Autodesk Fusion 360 part; units mm, degrees
sketch "Sketch1" plane through (0, 0, 0) normal (0, 0, 1) x (1, 0, 0)
  line L0 (0, 0) -> (100, 0)
  line L1 (100, 0) -> (100, 25)
  line L2 (100, 25) -> (0, 25)
  line L3 (0, 25) -> (0, 0)
  line L4 (0, 25) -> (100, 25)
  line L5 (100, 25) -> (100, 19)
  line L6 (100, 19) -> (0, 19)
  line L7 (0, 19) -> (0, 25)
  circle A0 centre (50, 10) radius 2
  circle A1 centre (10, 10) radius 2
  circle A2 centre (90, 10) radius 2
  dimension "d1" = 100
  dimension "d2" = 6
  dimension "d12" = 4
  dimension "d13" = 4
  dimension "d14" = 4
extrude "Extrude1" add sketch "Sketch1" along normal blind 4 contours L0 L1 L3 L6
extrude "Extrude2" add sketch "Sketch1" along normal blind 9 contours L1 L2 L3 L4 L5 L6 L7
sketch "Sketch2" plane through (0, 0, 9) normal (0, 0, 1) x (1, 0, 0)
  line L0 (0, 19) -> (100, 19)
  line L1 (100, 19) -> (100, 25)
  line L2 (100, 25) -> (0, 25)
  line L3 (0, 25) -> (0, 19)
  line L4 (0, 19) -> (100, 19)
  line L5 (100, 19) -> (100, 44)
  line L6 (100, 44) -> (0, 44)
  line L7 (0, 44) -> (0, 19)
  dimension "d7" = 25
  dimension "d8" = 100
extrude "Extrude3" add sketch "Sketch2" along normal blind 4
fillet "Fillet1" radius 2 13 edges at (50, 44, 13) (0, 31.5, 13) (100, 44, 11) (100, 31.5, 13) (50, 19, 13) (100, 19, 8.5) (100, 9.5, 4) (50, 0, 4) (0, 9.5, 4) (100, 0, 2) (0, 0, 2) (0, 19, 8.5) (0, 44, 11)
Could you check a few things on this model? Use its own coordinates, in mm. A direction names the side the tool comes from. Round coordinates to 2 decimals unless told otherwise and drop trailing zeros. Loops run counter-clockwise (first coordinate to the right, second up) from the corner with the lowest first, then second, coordinate; pieces in that order, holes last. Notation, with made-up numbers: (-33.5, -13) - (-20.5, -13) arc R20 ccw to (-20.5, 4) - close; hole circle Ø11 at (-22, -16). An arc over 180 degrees is marked (long way). Answer as CSV lines item,"result".
1. I want a section at A-A on x = 90. List the corners of the cut face in (y, z) for me.
Filled in:
outline,"(0, 0) - (8, 0) - (8, 4) - (2, 4) arc R2 ccw to (0, 2) - close; (12, 0) - (25, 0) - (25, 9) - (44, 9) - (44, 11) arc R2 ccw to (42, 13) - (21, 13) arc R2 ccw to (19, 11) - (19, 4) - (12, 4) - close"
2. I want a section at C-C on z = 1. List the corners of the cut face in (x, y) for me.
Filled in:
outline,"(0, 2) arc R2 ccw to (2, 0) - (98, 0) arc R2 ccw to (100, 2) - (100, 25) - (0, 25) - close; hole circle Ø4 at (10, 10); hole circle Ø4 at (50, 10); hole circle Ø4 at (90, 10)"
3. For pin 1 Ø2.5 at (x, y) = (90, 10) entering from -Z; pin 2 Ø4 at (x, z) = (28.5, 11.5) entering from -Y; pin 3 Ø15 at (x, y) = (26, 30) entering from -Z; pin 4 Ø5 at (x, y) = (62.5, 12.5) entering from +Z, each with a flat end and sliding along its axis, tell me the tip position at first contact or that it passes through.
Filled in:
pin 1,"passes through"
pin 2,"stops at y = 19"
pin 3,"stops at z = 0"
pin 4,"stops at z = 4"
4. We'd pull the mould along Y, two halves only. Please class faces 4 (the face through (99.4, 31.65, 12.43)), 5 (the face through (51.908, 9.399, 1.972)), 6 (the face through (0.57, 19.6, 7.56)): +Y half, -Y half, draft (parallel to the pull), parting line (faces both ways), or undercut.
Filled in:
face 4,"draft"
face 5,"undercut"
face 6,"-Y half"
5. On a 3-axis mill with a long thin cutter (end or side, diameter ignored), from which of +Z, -Z, +X, -X, +Y, -Y can I reach the whole of each face in a straight line? I mean faces 1 (the face through (99.4, 19.57, 7.56)), 2 (the face through (49, 0, 1)), 3 (the face through (49, 13, 4)). Say none if no direction works.
Filled in:
face 1,"+Z, +X, -Y"
face 2,"+Z, -Z, +X, -X, -Y"
face 3,"+Z, +X, -X, -Y"
6. Please list where these lines run through material, in increasing order: line 1 along Y through (x, z) = (50, 0.85); line 2 along Z through (x, y) = (9, 4); line 3 along Y through (x, z) = (95.5, 5). Write a range as [from, to].
Filled in:
line 1,"y = [0, 8], [12, 25]"
line 2,"z = [0, 4]"
line 3,"y = [19, 25]"
7. I want a section at D-D on z = 6.5. List the corners of the cut face in (x, y) for me.
Filled in:
outline,"(0, 21) arc R2 ccw to (2, 19) - (98, 19) arc R2 ccw to (100, 21) - (100, 25) - (0, 25) - close"
8. I want a section at B-B on y = 10. List the corners of the cut face in (x, z) for me, then the cut area to 3 significant figures.
Filled in:
outline,"(0, 0) - (8, 0) - (8, 4) - (2, 4) arc R2 ccw to (0, 2) - close; (12, 0) - (48, 0) - (48, 4) - (12, 4) - close; (52, 0) - (88, 0) - (88, 4) - (52, 4) - close; (92, 0) - (100, 0) - (100, 2) arc R2 ccw to (98, 4) - (92, 4) - close"
area,"350 mm^2"
